Build history of the part. All positions in model axes, mm. Round coordinates to 2 decimals unless told otherwise and drop trailing zeros. Write each loop counter-clockwise with the first axis right and the second up, starting at its lowest first coordinate (ties: lowest second). Pieces come first, ordered by that corner, then holes. Notation, with made-up numbers: M 51.25,62.25 L 60.25,62.25 A17 ccw 60.25,80.25 Z; hole C -15,-22 d1. An arc over 180 degrees is marked long. Write item = value, one per line.
from build123d import *

# Parameters (mm, degrees)
F0_W     = 63.5
F0_H     = 304.8
F1_DEPTH = 0.762
F2_R     = 3.937
F3_DEPTH = 12.7


with BuildPart() as f1:
    # F0 (on Front) → F1 (new body)
    with BuildSketch(Plane.XZ):
        Rectangle(F0_W, F0_H)
    extrude(amount=F1_DEPTH)

    # F2 (on Front) → F3 (cut, symmetric)
    with BuildSketch(Plane.XZ):
        with Locations((0, 127)):
            Circle(F2_R)
        with Locations((0, -127)):
            Circle(F2_R)
    extrude(amount=F3_DEPTH, both=True, mode=Mode.SUBTRACT)


solid = f1.part
1. Band-saw the part on B-B (x = 0). List the corners of the cut face in (y, z), plus the area to 3 significant figures.
Responses:
outline = M -0.76,-152.4 L 0,-152.4 L 0,-130.94 L -0.76,-130.94 Z; M -0.76,-123.06 L 0,-123.06 L 0,123.06 L -0.76,123.06 Z; M -0.76,130.94 L 0,130.94 L 0,152.4 L -0.76,152.4 Z
area = 220 mm²
2. Band-saw the part on A-A (z = -127). List the corners of the cut face in (x, y).
Responses:
outline = M -31.75,-0.76 L -3.94,-0.76 L -3.94,0 L -31.75,0 Z; M 3.94,-0.76 L 31.75,-0.76 L 31.75,0 L 3.94,0 Z
3. Mould opens along Z. For faces 1 (the face through (0, -0.762, 2)), 2 (the face through (-0.853, -0.376, 123.157)) say: pulls with the +Z half, pulls with the -Z half, needs draft (parallel to the pull), parting line crosses it, or undercut.
Responses:
face_1 = needs draft
face_2 = undercut
4. Probe probe 1 along Z at (x, y) = (0, -0.45); probe 2 along X at (y, z) = (-0.6, 127). List the from-to ranges inside material, lowest first.
Responses:
probe_1 = -152.4 to -130.94, -123.06 to 123.06, 130.94 to 152.4
probe_2 = -31.75 to -3.94, 3.94 to 31.75
